Part model, mm, in its own coordinate system. Coordinates: 2 decimals unless noted, no trailing zeros. Loops run counter-clockwise (first coordinate to the right, second up) from the corner with the lowest first, then second, coordinate; pieces in that order, holes last. Notation, with made-up numbers: (51, 87.5) - (106, 87.5) arc R14 cw to (106, 106.5) - close; hole circle Ø11 at (89, 15). An arc over 180 degrees is marked (long way). Use a Markdown table: item, result. Add a question column.
1) Band-saw the part on A-A (y = -8.5). Give the cut face in (x, z) (3 decimals), plus the area to 3 significant figures.
2) Pull direction X, two halves, no side cores. Call faces 1 (the face through (1, -38.1, 14)), 2 (the face through (-19.04, -22.49, 0.57)), 3 (the face through (27.74, -13.81, -14.1)), 4 (the face through (9.262, -3.625, 2.917)): +X half, -X half, draft (parallel to the pull), parting line (faces both ways), or undercut.
3) Band-saw the part on B-B (z = -2.5). Give the number of separate pieces and of enclosed holes in the cut face, plus the area to 3 significant figures.
4) Drop flat-ended pins along their axis: P1, Ø2, axis at x = 50, y = -12, coming from the +Z side; P2, Ø2, axis at x = 51, y = -6.5, coming from the -Z side; P3, Ø1, axis at x = 27, y = -22.5, coming from the +Z side; P4, Ø11.5, axis at x = 0, z = 0, coming from the -Y side. Give the stop position or say it passes through.
5) Probe probe 1 along Z at (x, y) = (4, -10); probe 2 along Z at (x, y) = (0, -17) (3 decimals); probe 3 along Z at (x, y) = (-14, -33). List the from-to ranges inside material, lowest first. Write a range as [from, to].
from build123d import *

# Parameters (mm, degrees)
F0_R     = 9.525
F0_R_2   = 6.35
F1_DEPTH = 25.4
F2_DEPTH = 38.1
F3_R     = 2.54


# Not quite as in the source:
# - a fillet or chamfer that OpenCascade refuses, or shapes differently, is made with other operations: its cross-section is extruded or revolved along the edge and cut away or added


with BuildPart() as f1:
    # F0 (on Front) → F1 (new body)
    with BuildSketch(Plane.XZ):
        with BuildLine():
            ThreePointArc((3.571875, -18.7121406842), (14.6790108446, -12.1420402167), (19.05, 0))
            ThreePointArc((19.05, 0), (14.6790108446, 12.1420402167), (3.571875, 18.7121406842))
            ThreePointArc((3.571875, 18.7121406842), (-19.05, 0), (3.571875, -18.7121406842))
        make_face()
        Circle(F0_R, mode=Mode.SUBTRACT)
        with BuildLine():
            ThreePointArc((3.571875, 18.7121406842), (14.6790108446, 12.1420402167), (19.05, 0))
            ThreePointArc((19.05, 0), (14.6790108446, -12.1420402167), (3.571875, -18.7121406842))
            Line((3.571875, -18.7121406842), (52.5859375, -9.3560703421))
            ThreePointArc((52.5859375, -9.3560703421), (41.275, 0), (52.5859375, 9.3560703421))
            Line((52.5859375, 9.3560703421), (3.571875, 18.7121406842))
        make_face()
        with BuildLine():
            ThreePointArc((60.325, 0), (58.1395054223, 6.0710201084), (52.5859375, 9.3560703421))
            ThreePointArc((52.5859375, 9.3560703421), (41.275, 0), (52.5859375, -9.3560703421))
            ThreePointArc((52.5859375, -9.3560703421), (58.1395054223, -6.0710201084), (60.325, 0))
        make_face()
        with Locations((50.8, 0)):
            Circle(F0_R_2, mode=Mode.SUBTRACT)
    extrude(amount=F1_DEPTH)

    # F0 (on Front) → F2 (join)
    with BuildSketch(Plane.XZ):
        with BuildLine():
            ThreePointArc((3.571875, -18.7121406842), (14.6790108446, -12.1420402167), (19.05, 0))
            ThreePointArc((19.05, 0), (14.6790108446, 12.1420402167), (3.571875, 18.7121406842))
            ThreePointArc((3.571875, 18.7121406842), (-19.05, 0), (3.571875, -18.7121406842))
        make_face()
        Circle(F0_R, mode=Mode.SUBTRACT)
    extrude(amount=F2_DEPTH)

    # F3
    f3_edges = [f1.edges().sort_by_distance(p)[0] for p in [
        (28.078906, 0, -14.034106),
        (-3.571875, -38.1, 18.712141),
    ]]
    fillet(f3_edges, radius=F3_R)

    # F4: chamfer of 3.81 on 4 edges, made by hand

    # F4_s1 → F4_t2 (revolve, cut)
    with BuildSketch(Plane.XY):
        Polygon((13.335, -38.1), (9.525, -34.29), (9.525, -38.1), align=None)
    revolve(axis=Axis((0, -38.1, 0), (0, -1, 0)), mode=Mode.SUBTRACT)

    # F4_s3 → F4_t4 (revolve, cut)
    with BuildSketch(Plane.XY):
        Polygon((60.96, -25.4), (57.15, -21.59), (57.15, -25.4), align=None)
    revolve(axis=Axis((50.8, -25.4, 0), (0, -1, 0)), mode=Mode.SUBTRACT)

    # F4_s5 → F4_t6 (revolve, cut)
    with BuildSketch(Plane.XY):
        Polygon((13.335, 0), (9.525, -3.81), (9.525, 0), align=None)
    revolve(axis=Axis((0, 0, 0), (0, -1, 0)), mode=Mode.SUBTRACT)

    # F4_s7 → F4_t8 (revolve, cut)
    with BuildSketch(Plane.XY):
        Polygon((60.96, 0), (57.15, -3.81), (57.15, 0), align=None)
    revolve(axis=Axis((50.8, 0, 0), (0, -1, 0)), mode=Mode.SUBTRACT)


solid = f1.part
Answer block:
| question | item | result |
|---|---|---|
| 1 | outline | (3.572, -18.712) - (52.586, -9.356) arc R9.525 ccw to (52.586, 9.356) - (3.572, 18.712) arc R19.05 ccw (long way) to start; hole circle Ø19.05 at (0, 0); hole circle Ø12.7 at (50.8, 0) |
| 1 | area | 1,780 mm2 |
| 2 | face 1 | draft |
| 2 | face 2 | parting line |
| 2 | face 3 | +X half |
| 2 | face 4 | undercut |
| 3 | separate pieces | 3 |
| 3 | enclosed holes | 0 |
| 3 | area | 1,420 mm2 |
| 4 | P1 | z = 10.04 |
| 4 | P2 | z = -9.85 |
| 4 | P3 | z = 14.34 |
| 4 | P4 | through |
| 5 | probe 1 | [-18.63, -8.64], [8.64, 18.63] |
| 5 | probe 2 | [-19.05, -9.525], [9.525, 19.05] |
| 5 | probe 3 | [-12.92, 12.92] |
